Job drawing, mm, ordinate dimensions from the low corner. One solid piece. A direction names the side the tool comes from. Round coordinates to 2 decimals unless told otherwise and drop trailing zeros. Write each loop counter-clockwise with the first axis right and the second up, starting at its lowest first coordinate (ties: lowest second). Pieces come first, ordered by that corner, then holes. Notation, with made-up numbers: (81, -18) - (140, -18) arc R24 ccw to (140, 6) - close; hole circle Ø2 at (-9, -16.5). An arc over 180 degrees is marked (long way). Write each question's results on one line, items separated by ' | '.
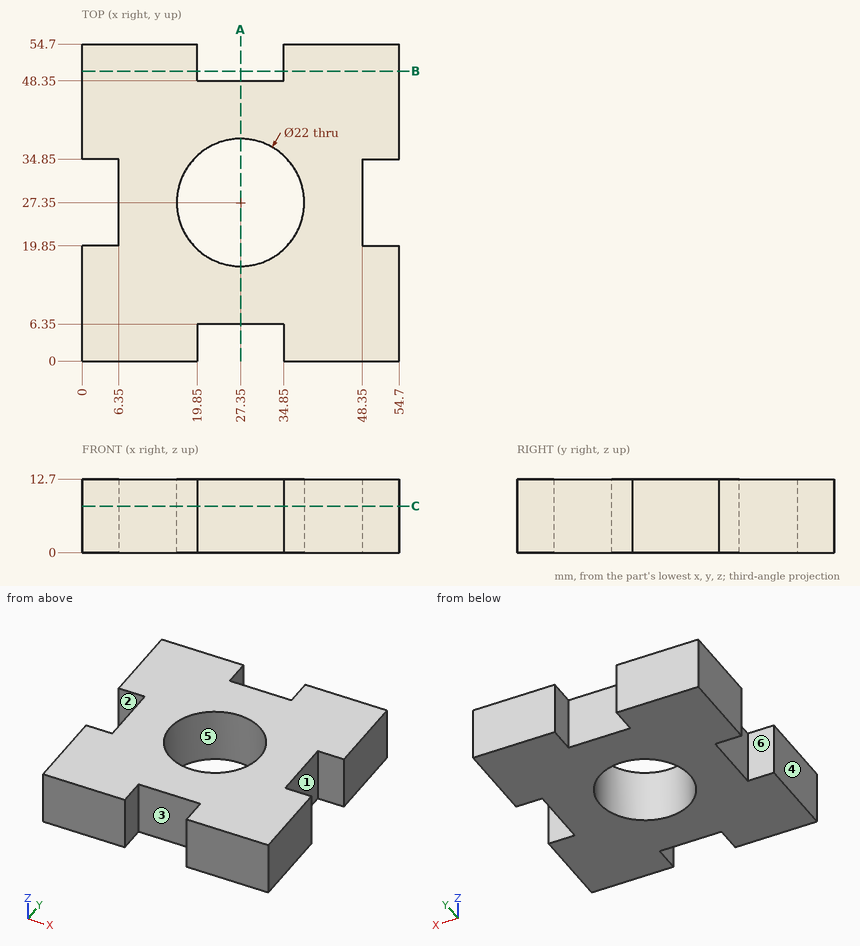
(1) Slice it at C-C, the plane z = 8. Write the cut outline in (x, y), and give its area (3 significant figures).
Worked answers:
outline: (0, 0) - (19.85, 0) - (19.85, 6.35) - (34.85, 6.35) - (34.85, 0) - (54.7, 0) - (54.7, 19.85) - (48.35, 19.85) - (48.35, 34.85) - (54.7, 34.85) - (54.7, 54.7) - (34.85, 54.7) - (34.85, 48.35) - (19.85, 48.35) - (19.85, 54.7) - (0, 54.7) - (0, 34.85) - (6.35, 34.85) - (6.35, 19.85) - (0, 19.85) - close; hole circle Ø22 at (27.35, 27.35) | area: 2,230 mm2
(2) Flat gauge pins, fed straight in: pin 1 Ø1.9 at (x, z) = (3, 6.5) entering from -Y; pin 2 Ø4 at (x, z) = (23.5, 7.5) entering from -Y; pin 3 Ø6.5 at (y, z) = (25.5, 8) entering from +X. Where does each tip first touch, or does it go through?
Worked answers:
pin 1: stops at y = 0 | pin 2: stops at y = 6.35 | pin 3: stops at x = 48.35
(3) Drill centre lines: probe 1 along Y at (x, z) = (27.35, 9); probe 2 along X at (y, z) = (4.5, 10.75); probe 3 along X at (y, z) = (32, 0.75). Where is each one in solid material? Low to high. Write a range as [from, to].
Worked answers:
probe 1: y = [6.35, 16.35], [38.35, 48.35] | probe 2: x = [0, 19.85], [34.85, 54.7] | probe 3: x = [6.35, 17.38], [37.32, 48.35]
(4) Tool access for the marked faces 1, 2 and 3: list every direction of +Z, -Z, +X, -X, +Y, -Y with a clear straight run to the whole face (end or side of a thin tool).
Worked answers:
face 1: +Z, -Z, +X | face 2: +Z, -Z, -X | face 3: +Z, -Z, -Y
(5) Two-plate mould, pull along X, no slides. Class the marked faces 4, 5 and 6: released by +X, released by -X, zero draft, split by the parting line, or undercut.
Worked answers:
face 4: released by -X | face 5: undercut | face 6: zero draft
(6) Slice it at A-A, the plane x = 27.35. Write the cut outline in (y, z).
Worked answers:
outline: (6.35, 0) - (16.35, 0) - (16.35, 12.7) - (6.35, 12.7) - close; (38.35, 0) - (48.35, 0) - (48.35, 12.7) - (38.35, 12.7) - close
(7) Slice it at B-B, the plane y = 50. Write the cut outline in (x, z).
Worked answers:
outline: (0, 0) - (19.85, 0) - (19.85, 12.7) - (0, 12.7) - close; (34.85, 0) - (54.7, 0) - (54.7, 12.7) - (34.85, 12.7) - close
